Verification items for the finished model (mm, model axes). Face numbers are marked on the shaded views. A direction names the side the tool comes from. Round coordinates to 2 decimals unless told otherwise and drop trailing zeros. Order: outer loops, then holes, each group sorted by start corner. A loop starts at its lowest first (then second) coordinate and runs counter-clockwise, first axis right, second up. Notation, with made-up numbers: (71, -26) -> (111, -26) arc R31 cw to (111, 0) -> close; hole circle Ø9 at (4, 8.5). An arc over 180 degrees is marked (long way). Return JSON: item names as keys, results as strings. Group by question number.
1) Tool access check on the marked faces 1 and 2. Record the directions out of +Z, -Z, +X, -X, +Y, -Y that give a thin tool (end or side, any length) a straight path to the whole face; none if there is none.
2) Section check A-A on z = -17. Enter the section's corners in (x, y), plus the area to 3 significant figures.
3) Section check D-D on y = 30. Enter the section's corners in (x, z).
4) Scan lines: L1, parallel to Y at x = 23, z = -17; L2, parallel to Z at x = 20, y = 18; L3, parallel to Z at x = 20, y = 46. Record each from-to range of solid material in increasing order.
5) Draft check along Z on the marked faces 3, 4 and 5. Enter one of: pulls with the +Z half, pulls with the -Z half, needs draft (parallel to the pull), parting line crosses it, or undercut.
6) Section check C-C on x = 16.5. State how many separate pieces and enclosed holes the cut face has, plus the area to 3 significant figures.
7) Section check B-B on y = 18. Enter the section's corners in (x, z).
8) Depth check by flat-ended pin: pin 1 (24 mm diameter, centred on y = 18, z = -17, fed in from -X); pin 2 (1.1 mm diameter, centred on x = 39.5, z = -33, fed in from -Y); pin 3 (1 mm diameter, centred on x = 23, z = -31, fed in from +Y). Enter the tip coordinate at first touch or a pass-through.
```python
from build123d import *

# Parameters (mm, degrees)
BOSS_EXTRUDE1_DEPTH = 36
SKETCH2_R           = 7.5
CUT_EXTRUDE1_DEPTH  = 72.449282712
BOSS_EXTRUDE5_DEPTH = 7
SKETCH9_W           = 40.098560475
SKETCH9_H           = 15
BOSS_EXTRUDE6_DEPTH = 18
FILLET4_R           = 11


with BuildPart() as part:
    # Sketch1 → Boss-Extrude1 (new body)
    with BuildSketch(Plane(origin=(0, 0, 0), x_dir=(1, 0, 0), z_dir=(0, 1, 0))):
        Polygon((27.5, 0), (12.5, 0), (17.5, 34), (0, 47), (40, 47), (22.5, 34), align=None)
    extrude(amount=BOSS_EXTRUDE1_DEPTH)

    # Sketch2 → Cut-Extrude1 (cut, through all)
    with BuildSketch(Plane(origin=(0, 0, 0), x_dir=(0, 0, -1), z_dir=(1, 0, 0))):
        with Locations(Location((17, 18, 0), (0, 0, 180))):
            Circle(SKETCH2_R)
    extrude(amount=CUT_EXTRUDE1_DEPTH, mode=Mode.SUBTRACT)

    # Sketch7 → Boss-Extrude5 (add)
    with BuildSketch(Plane(origin=(0, 36, 0), x_dir=(1, 0, 0), z_dir=(0, 1, 0))):
        Polygon((0, 47), (40, 47), (22.5, 34), (22.794117647, 32), (17.205882353, 32), (17.5, 34), align=None)
    extrude(amount=BOSS_EXTRUDE5_DEPTH)

    # Sketch9 → Boss-Extrude6 (add)
    with BuildSketch(Plane(origin=(0, 43, 0), x_dir=(1, 0, 0), z_dir=(0, 1, 0))):
        with Locations((20.049280237, 39.5)):
            Rectangle(SKETCH9_W, SKETCH9_H)
    extrude(amount=BOSS_EXTRUDE6_DEPTH)

    # Fillet4
    fillet4_edges = [part.edges().sort_by_distance(p)[0] for p in [
        (31.25, 43, -40.5),
        (8.75, 43, -40.5),
    ]]
    fillet(fillet4_edges, radius=FILLET4_R)


solid = part.part
```
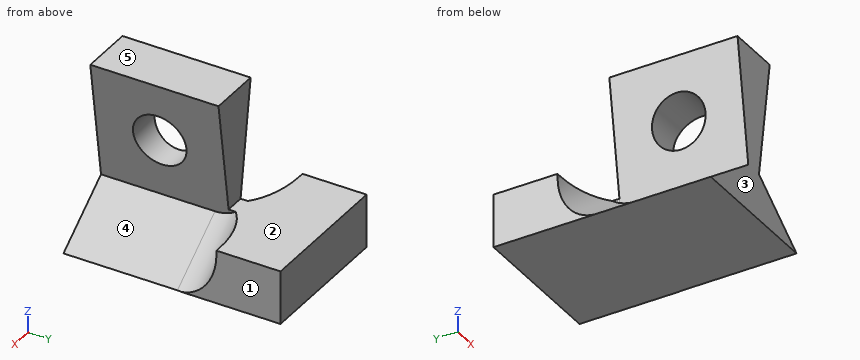
Check result:
{
 "1": {"face 1": "+Z, -Z, +X, +Y, -Y", "face 2": "+Z, +X, -X, +Y"},
 "2": {"outline": "(15, 0) -> (25, 0) -> (25, 10.5) -> (15, 10.5) -> close; (15, 25.5) -> (25, 25.5) -> (25, 36) -> (15, 36) -> close", "area": "210 mm^2"},
 "3": {"outline": "(0, -47) -> (40, -47) -> (22.5, -34) -> (27.5, 0) -> (12.5, 0) -> (17.5, -34) -> close"},
 "4": {"L1": "0 to 10.5, 25.5 to 36", "L2": "-47 to -24.5, -9.5 to 0", "L3": "-47 to -32"},
 "5": {"face 3": "needs draft", "face 4": "undercut", "face 5": "pulls with the +Z half"},
 "6": {"separate pieces": "2", "enclosed holes": "1", "area": "1,620 mm^2"},
 "7": {"outline": "(0, -47) -> (40, -47) -> (22.5, -34) -> (23.9, -24.5) -> (16.1, -24.5) -> (17.5, -34) -> close; (12.5, 0) -> (13.9, -9.5) -> (26.1, -9.5) -> (27.5, 0) -> close"},
 "8": {"pin 1": "x = 13.24", "pin 2": "y = 42.98", "pin 3": "y = 36"}
}
